Could you check a few things on this model? Use its own coordinates, in mm. A direction names the side the tool comes from. Round coordinates to 2 decimals unless told otherwise and drop trailing zeros. Loops run counter-clockwise (first coordinate to the right, second up) from the corner with the lowest first, then second, coordinate; pieces in that order, holes last. Notation, with made-up numbers: (12.5, 67) -> (58.5, 67) arc R25 ccw to (58.5, 80) -> close; hole circle Ø5 at (68.5, -10). An arc over 180 degrees is marked (long way). Write each question's results on one line, items separated by ' | '.
from build123d import *

# Parameters (mm, degrees)
SKETCH3_W                                      = 180
SKETCH3_H                                      = 90
BOSS_EXTRUDE3_DEPTH                            = 3
SKETCH4_W                                      = 8.5
SKETCH4_H                                      = 61.5
CUT_EXTRUDE1_DEPTH                             = 3
CSK_FOR_M5_FLAT_HEAD_MACHINE_SCREW1_AT_2_COUNT = 2
CSK_FOR_M5_FLAT_HEAD_MACHINE_SCREW1_AT_2_PITCH = 167.524625056
CSK_FOR_M5_FLAT_HEAD_MACHINE_SCREW1_AT_3_COUNT = 2
CSK_FOR_M5_FLAT_HEAD_MACHINE_SCREW1_AT_3_PITCH = 71.5
CSK_FOR_M5_FLAT_HEAD_MACHINE_SCREW1_AT_4_COUNT = 2
CSK_FOR_M5_FLAT_HEAD_MACHINE_SCREW1_AT_4_PITCH = 151.5
CSK_SLOT_FOR_M5_FLAT_HEAD_MACHINE_SCREW1_DEPTH = 3
SKETCH12_W                                     = 9.5
SKETCH12_H                                     = 10
BOSS_EXTRUDE4_DEPTH                            = 10
CSK_FOR_M4_SFHCS1_D                            = 4.5
CSK_FOR_M4_SFHCS1_DEPTH                        = 10
CSK_FOR_M4_SFHCS1_CSINK_D                      = 8.96
CSK_FOR_M4_SFHCS1_CSINK_ANGLE                  = 90
M4X0_7_TAPPED_HOLE1_D                          = 3.3
BOSS_EXTRUDE5_DEPTH                            = 14


with BuildPart() as part:
    # Sketch3 → Boss-Extrude3 (new body)
    with BuildSketch(Plane.XY):
        Rectangle(SKETCH3_W, SKETCH3_H)
    extrude(amount=BOSS_EXTRUDE3_DEPTH)

    # Sketch4 → Cut-Extrude1 (cut)
    with BuildSketch(Plane.XY.offset(3)):
        with BuildLine():
            Line((-4.25, -30.75), (-4.25, 30.75))
            ThreePointArc((-4.25, 30.75), (-7.785533906, 32.214466094), (-9.25, 35.75))
            Line((-9.25, 35.75), (-70.75, 35.75))
            ThreePointArc((-70.75, 35.75), (-72.214466094, 32.214466094), (-75.75, 30.75))
            Line((-75.75, 30.75), (-75.75, -30.75))
            ThreePointArc((-75.75, -30.75), (-72.214466094, -32.214466094), (-70.75, -35.75))
            Line((-70.75, -35.75), (-9.25, -35.75))
            ThreePointArc((-9.25, -35.75), (-7.785533906, -32.214466094), (-4.25, -30.75))
        make_face()
        Rectangle(SKETCH4_W, SKETCH4_H)
        with BuildLine():
            ThreePointArc((9.25, 35.75), (7.785533906, 32.214466094), (4.25, 30.75))
            Line((4.25, 30.75), (4.25, -30.75))
            ThreePointArc((4.25, -30.75), (7.785533906, -32.214466094), (9.25, -35.75))
            Line((9.25, -35.75), (70.75, -35.75))
            ThreePointArc((70.75, -35.75), (72.214466094, -32.214466094), (75.75, -30.75))
            Line((75.75, -30.75), (75.75, 30.75))
            ThreePointArc((75.75, 30.75), (72.214466094, 32.214466094), (70.75, 35.75))
            Line((70.75, 35.75), (9.25, 35.75))
        make_face()
    extrude(amount=-CUT_EXTRUDE1_DEPTH, mode=Mode.SUBTRACT)

    # Sketch8 → CSK for M5 Flat Head Machine Screw1 (revolve, cut)
    with BuildSketch(Plane(origin=(-75.75, 35.75, 3), x_dir=(0, -1, 0), z_dir=(1, 0, 0))):
        Polygon((0, 0), (0, 3), (2.55, 3), (2.55, 0.85), (3.4, 0), align=None)
    csk_for_m5_flat_head_machine_screw1 = revolve(axis=Axis((-75.75, 35.75, 9.35), (0, 0, -1)), mode=Mode.SUBTRACT)

    # CSK for M5 Flat Head Machine Screw1 at 2: CSK for M5 Flat Head Machine Screw1 ×2
    with Locations(*[Vector(0.9043446594777974, -0.4268029251000826, 0) * (i * CSK_FOR_M5_FLAT_HEAD_MACHINE_SCREW1_AT_2_PITCH) for i in range(1, CSK_FOR_M5_FLAT_HEAD_MACHINE_SCREW1_AT_2_COUNT)]):
        add(csk_for_m5_flat_head_machine_screw1, mode=Mode.SUBTRACT)

    # CSK for M5 Flat Head Machine Screw1 at 3: CSK for M5 Flat Head Machine Screw1 ×2
    with Locations(*[(0, -i * CSK_FOR_M5_FLAT_HEAD_MACHINE_SCREW1_AT_3_PITCH, 0) for i in range(1, CSK_FOR_M5_FLAT_HEAD_MACHINE_SCREW1_AT_3_COUNT)]):
        add(csk_for_m5_flat_head_machine_screw1, mode=Mode.SUBTRACT)

    # CSK for M5 Flat Head Machine Screw1 at 4: CSK for M5 Flat Head Machine Screw1 ×2
    with Locations(*[(i * CSK_FOR_M5_FLAT_HEAD_MACHINE_SCREW1_AT_4_PITCH, 0, 0) for i in range(1, CSK_FOR_M5_FLAT_HEAD_MACHINE_SCREW1_AT_4_COUNT)]):
        add(csk_for_m5_flat_head_machine_screw1, mode=Mode.SUBTRACT)

    # CSK SLOT for M5 Flat Head Machine Screw1: read off the stored shape, not the designer's step
    # CSK SLOT for M5 Flat Head Machine Sc 2 → CSK SLOT for M5 Flat Head Machine Screw1 (cut)
    with BuildSketch(Plane.XY):
        with BuildLine():
            Line((-4.25, 33.2), (4.25, 33.2))
            ThreePointArc((4.25, 33.2), (6.8, 35.75), (4.25, 38.3))
            Line((4.25, 38.3), (-4.25, 38.3))
            ThreePointArc((-4.25, 38.3), (-6.8, 35.75), (-4.25, 33.2))
        make_face()
        with BuildLine():
            Line((-4.25, -38.3), (4.25, -38.3))
            ThreePointArc((4.25, -38.3), (6.8, -35.75), (4.25, -33.2))
            Line((4.25, -33.2), (-4.25, -33.2))
            ThreePointArc((-4.25, -33.2), (-6.8, -35.75), (-4.25, -38.3))
        make_face()
    extrude(amount=CSK_SLOT_FOR_M5_FLAT_HEAD_MACHINE_SCREW1_DEPTH, mode=Mode.SUBTRACT)

    # CSK SLOT for M5 Flat Head Machine Sc 3: loft between two sections, ruled curve by curve
    csk_slot_for_m5_flat_head_machine_sc_3_from = [
        Edge.make_three_point_arc((4.25, 33.2, 2.15), (6.053122292, 33.946877708, 2.15), (6.8, 35.75, 2.15)),
        Edge.make_three_point_arc((6.8, 35.75, 2.15), (6.053122292, 37.553122292, 2.15), (4.25, 38.3, 2.15)),
        Edge.make_three_point_arc((-4.25, 38.3, 2.15), (-6.053122292, 37.553122292, 2.15), (-6.8, 35.75, 2.15)),
        Edge.make_three_point_arc((-6.8, 35.75, 2.15), (-6.053122292, 33.946877708, 2.15), (-4.25, 33.2, 2.15)),
        Edge.make_line((4.25, 38.3, 2.15), (-4.25, 38.3, 2.15)),
        Edge.make_line((4.25, 33.2, 2.15), (-4.25, 33.2, 2.15)),
    ]
    csk_slot_for_m5_flat_head_machine_sc_3_to = [
        Edge.make_three_point_arc((4.25, 32.35, 3), (6.654163056, 33.345836944, 3), (7.65, 35.75, 3)),
        Edge.make_three_point_arc((7.65, 35.75, 3), (6.654163056, 38.154163056, 3), (4.25, 39.15, 3)),
        Edge.make_three_point_arc((-4.25, 39.15, 3), (-6.654163056, 38.154163056, 3), (-7.65, 35.75, 3)),
        Edge.make_three_point_arc((-7.65, 35.75, 3), (-6.654163056, 33.345836944, 3), (-4.25, 32.35, 3)),
        Edge.make_line((4.25, 39.15, 3), (-4.25, 39.15, 3)),
        Edge.make_line((4.25, 32.35, 3), (-4.25, 32.35, 3)),
    ]
    csk_slot_for_m5_flat_head_machine_sc_3 = Solid(Shell([*[Face.make_surface_from_curves(csk_slot_for_m5_flat_head_machine_sc_3_from[k], csk_slot_for_m5_flat_head_machine_sc_3_to[k]) for k in range(6)], Face(Wire(csk_slot_for_m5_flat_head_machine_sc_3_from)), Face(Wire(csk_slot_for_m5_flat_head_machine_sc_3_to))]))
    add(csk_slot_for_m5_flat_head_machine_sc_3, mode=Mode.SUBTRACT)

    # CSK SLOT for M5 Flat Head Machine Sc 4: loft between two sections, ruled curve by curve
    csk_slot_for_m5_flat_head_machine_sc_4_from = [
        Edge.make_three_point_arc((4.25, -38.3, 2.15), (6.053122292, -37.553122292, 2.15), (6.8, -35.75, 2.15)),
        Edge.make_three_point_arc((6.8, -35.75, 2.15), (6.053122292, -33.946877708, 2.15), (4.25, -33.2, 2.15)),
        Edge.make_three_point_arc((-4.25, -33.2, 2.15), (-6.053122292, -33.946877708, 2.15), (-6.8, -35.75, 2.15)),
        Edge.make_three_point_arc((-6.8, -35.75, 2.15), (-6.053122292, -37.553122292, 2.15), (-4.25, -38.3, 2.15)),
        Edge.make_line((4.25, -33.2, 2.15), (-4.25, -33.2, 2.15)),
        Edge.make_line((4.25, -38.3, 2.15), (-4.25, -38.3, 2.15)),
    ]
    csk_slot_for_m5_flat_head_machine_sc_4_to = [
        Edge.make_three_point_arc((4.25, -39.15, 3), (6.654163056, -38.154163056, 3), (7.65, -35.75, 3)),
        Edge.make_three_point_arc((7.65, -35.75, 3), (6.654163056, -33.345836944, 3), (4.25, -32.35, 3)),
        Edge.make_three_point_arc((-4.25, -32.35, 3), (-6.654163056, -33.345836944, 3), (-7.65, -35.75, 3)),
        Edge.make_three_point_arc((-7.65, -35.75, 3), (-6.654163056, -38.154163056, 3), (-4.25, -39.15, 3)),
        Edge.make_line((4.25, -32.35, 3), (-4.25, -32.35, 3)),
        Edge.make_line((4.25, -39.15, 3), (-4.25, -39.15, 3)),
    ]
    csk_slot_for_m5_flat_head_machine_sc_4 = Solid(Shell([*[Face.make_surface_from_curves(csk_slot_for_m5_flat_head_machine_sc_4_from[k], csk_slot_for_m5_flat_head_machine_sc_4_to[k]) for k in range(6)], Face(Wire(csk_slot_for_m5_flat_head_machine_sc_4_from)), Face(Wire(csk_slot_for_m5_flat_head_machine_sc_4_to))]))
    add(csk_slot_for_m5_flat_head_machine_sc_4, mode=Mode.SUBTRACT)

    # Sketch12 → Boss-Extrude4 (add)
    with BuildSketch(Plane(origin=(0, 0, 0), x_dir=(-1, 0, 0), z_dir=(0, 0, -1))):
        with Locations((-85.25, 40)):
            Rectangle(SKETCH12_W, SKETCH12_H)
        with Locations((-85.25, -40)):
            Rectangle(SKETCH12_W, SKETCH12_H)
    boss_extrude4 = extrude(amount=BOSS_EXTRUDE4_DEPTH)

    # CSK for M4 SFHCS1
    with Locations(Plane(origin=(0, -35, 0), x_dir=(1, 0, 0), z_dir=(0, 1, 0))):
        with Locations((85.162636167, 5)):
            csk_for_m4_sfhcs1 = CounterSinkHole(CSK_FOR_M4_SFHCS1_D / 2, CSK_FOR_M4_SFHCS1_CSINK_D / 2, depth=CSK_FOR_M4_SFHCS1_DEPTH, counter_sink_angle=CSK_FOR_M4_SFHCS1_CSINK_ANGLE)

    # M4x0.7 Tapped Hole1 (through all)
    with Locations(Plane(origin=(0, 45, 0), x_dir=(1, 0, 0), z_dir=(0, 1, 0))):
        with Locations((85.25, 5)):
            m4x0_7_tapped_hole1 = Hole(M4X0_7_TAPPED_HOLE1_D / 2)

    # Mirror1: Boss-Extrude4, CSK for M4 SFHCS1, M4x0.7 Tapped Hole1 across plane
    add(boss_extrude4.mirror(Plane(origin=(0, 0, 0), x_dir=(0, 0, 1), z_dir=(1, 0, 0))))
    add(csk_for_m4_sfhcs1.mirror(Plane(origin=(0, 0, 0), x_dir=(0, 0, 1), z_dir=(1, 0, 0))), mode=Mode.SUBTRACT)
    add(m4x0_7_tapped_hole1.mirror(Plane(origin=(0, 0, 0), x_dir=(0, 0, 1), z_dir=(1, 0, 0))), mode=Mode.SUBTRACT)

    # Sketch20 → Boss-Extrude5 (add)
    with BuildSketch(Plane.ZY.offset(90)):
        Polygon((3, -45), (3, 45), (-10, 45), (-10, 35), (0, 35), (0, -35), (-10, -35), (-10, -45), align=None)
    extrude(amount=BOSS_EXTRUDE5_DEPTH)


solid = part.part
1) If we mould it in two halves opening along X, with no side actions, what happens to faces 1 (the flat face through (-104, 1, 1)), 2 (the flat face through (88.44, -35, -8.31)), 3 (the cylindrical face through (-72.25, -32.18, 1.52))? For each: released by +X, released by -X, zero draft, split by the parting line, or undercut.
Model answer:
face 1: released by -X | face 2: zero draft | face 3: undercut
2) For faces 4 (the cylindrical face through (87.41, -41.17, -5.1)), 5 (the flat face through (83, 35, -5)), 6 (the flat face through (80.5, 40, -5)), 7 (the cylindrical face through (72.18, -32.25, 1.52)), which set-ups out of +Z, -Z, +X, -X, +Y, -Y let a thin tool reach every point of the face, with its end or its side?
Model answer:
face 4: -Y | face 5: -Z, +X, -X | face 6: -Z, +Y, -Y | face 7: +Z, -Z
3) I need wall thicknesses on line 1 (X direction, y = 33.5, z = 1.25); line 2 (Y direction, x = -4, z = 0.25); line 3 (X direction, y = -36, z = -1). Which ranges of each line are inside material? Lowest first, please.
Model answer:
line 1: x = -104 to -76.95, -74.55 to -71.28, -8.72 to -5.45, 5.45 to 8.72, 71.28 to 74.55, 76.95 to 90 | line 2: y = -45 to -38.3, -33.2 to -30.75, 30.75 to 33.2, 38.3 to 45 | line 3: x = -104 to -80.5, 80.5 to 90
4) I'm going to push flat-ended pins straight in: pin 1 (3 mm diameter, centred on x = -75.75, y = 35.75, fed in from -Z); pin 2 (6 mm diameter, centred on x = 75.75, y = -35.75, fed in from +Z). Where does each tip first touch, or does it pass through?
Model answer:
pin 1: passes through | pin 2: stops at z = 2.6
5) I want a section at A-A, the plane x = 24.5. Write out the boundary of the cut face in (y, z).
Model answer:
outline: (-45, 0) -> (-35.75, 0) -> (-35.75, 3) -> (-45, 3) -> close; (35.75, 0) -> (45, 0) -> (45, 3) -> (35.75, 3) -> close
6) I want a section at B-B, the plane y = 20. Write out the boundary of the cut face in (x, z).
Model answer:
outline: (-104, 0) -> (-75.75, 0) -> (-75.75, 3) -> (-104, 3) -> close; (75.75, 0) -> (90, 0) -> (90, 3) -> (75.75, 3) -> close
